Here's how the part is built. I have some questions about the finished solid (model axes, mm). Round coordinates to 2 decimals unless told otherwise and drop trailing zeros. Write each loop counter-clockwise with the first axis right and the second up, starting at its lowest first coordinate (ties: lowest second). Pieces come first, ordered by that corner, then holes. Notation, with made-up numbers: M -19,34.5 L -14,34.5 A25 ccw -14,62.5 Z; hole C 10,26.5 d5. An arc over 180 degrees is marked long. Write item = value, one per line. Start each with the question number.
(1) I want a section at A-A (z = 6). List the corners of the cut face in (x, y) for me, and give its area (3 significant figures).
(2) I want a section at B-B (x = 31.5). List the corners of the cut face in (y, z) for me, and give its area (3 significant figures).
(3) I need wall thicknesses on line 1 along Y through (x, z) = (9.5, 6); line 2 along Y through (x, z) = (37, 6.5); line 3 along Z through (x, y) = (3, 21.5). Which ranges of each line are inside material? Lowest first, please.
(4) I want a section at C-C (y = 5). List the corners of the cut face in (x, z) for me, and give its area (3 significant figures).
(5) I want a section at D-D (y = 19). List the corners of the cut face in (x, z) for me.
```python
from build123d import *

# Parameters (mm, degrees)
ESQUISSE1_W                       = 40
ESQUISSE1_H                       = 25
BOSS_EXTRU_1_DEPTH                = 12
DIAM_TRE_DU_PER_AGE_4_0_4_1_D     = 4
DIAM_TRE_DU_PER_AGE_4_0_4_1_DEPTH = 40


with BuildPart() as part:
    # Esquisse1 → Boss.-Extru.1 (new body)
    with BuildSketch(Plane.XY):
        with Locations((20, 12.5)):
            Rectangle(ESQUISSE1_W, ESQUISSE1_H)
    extrude(amount=BOSS_EXTRU_1_DEPTH)

    # Diamètre du perçage Ø4.0 (4)1
    with Locations(Plane(origin=(40, 0, 0), x_dir=(0, 0, -1), z_dir=(1, 0, 0))):
        with Locations((-6, 20), (-6, 5)):
            Hole(DIAM_TRE_DU_PER_AGE_4_0_4_1_D / 2, depth=DIAM_TRE_DU_PER_AGE_4_0_4_1_DEPTH)


solid = part.part
```
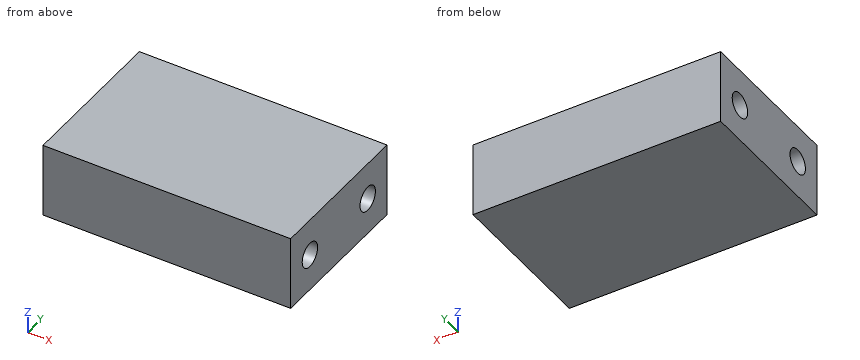
Returned:
q1.outline = M 0,0 L 40,0 L 40,3 L 0,3 Z; M 0,7 L 40,7 L 40,18 L 0,18 Z; M 0,22 L 40,22 L 40,25 L 0,25 Z
q1.area = 680 mm²
q2.outline = M 0,0 L 25,0 L 25,12 L 0,12 Z; hole C 5,6 d4; hole C 20,6 d4
q2.area = 275 mm²
q3.line_1 = 0 to 3, 7 to 18, 22 to 25
q3.line_2 = 0 to 3.06, 6.94 to 18.06, 21.94 to 25
q3.line_3 = 0 to 4.68, 7.32 to 12
q4.outline = M 0,0 L 40,0 L 40,4 L 0,4 Z; M 0,8 L 40,8 L 40,12 L 0,12 Z
q4.area = 320 mm²
q5.outline = M 0,0 L 40,0 L 40,4.27 L 0,4.27 Z; M 0,7.73 L 40,7.73 L 40,12 L 0,12 Z
